from build123d import *

# Parameters (mm, degrees)
TIGE_START              = -12
ESQUISSE1_R             = 2
TIGE_DEPTH              = 12
CHANFREIN_D_ENTR_E_SIZE = 0.7
HEXAGONE_DEPTH          = 2


with BuildPart() as part:
    # Esquisse1 → Tige (new body)
    with BuildSketch(Plane(origin=(0, 0, 0), x_dir=(1, 0, 0), z_dir=(0, 1, 0)).offset(TIGE_START)):
        with Locations(Location((0, 0, 0), (0, 0, 270))):
            Circle(ESQUISSE1_R)
    extrude(amount=TIGE_DEPTH)

    # Chanfrein d'entrée
    chanfrein_d_entr_e_edges = [part.edges().sort_by_distance(p)[0] for p in [
        (0, -12, -2),
    ]]
    chamfer(chanfrein_d_entr_e_edges, length=CHANFREIN_D_ENTR_E_SIZE)

    # Esquisse2 → Tête (revolve)
    with BuildSketch(Plane.XY, mode=Mode.PRIVATE) as t_te_sk:
        with BuildLine():
            Line((1.5, 4), (1.5, 2))
            Line((1.5, 2), (0, 1.133974596))
            Line((0, 1.133974596), (0, 0))
            Line((0, 0), (3.5, 0))
            Line((3.5, 0), (3.5, 3.6))
            ThreePointArc((3.5, 3.6), (3.382842712, 3.882842712), (3.1, 4))
            Line((3.1, 4), (1.5, 4))
        make_face()
    revolve(t_te_sk.sketch.rotate(Axis((0, 4, 0), (0, -1, 0)), 180), axis=Axis((0, 4, 0), (0, -1, 0)))

    # Esquisse3 → Hexagone (cut)
    with BuildSketch(Plane(origin=(0, 4, -3), x_dir=(1, 0, 0), z_dir=(0, -1, 0))):
        Polygon((0.866025404, 4.5), (-0.866025404, 4.5), (-1.732050808, 3), (-0.866025404, 1.5), (0.866025404, 1.5), (1.732050808, 3), align=None)
    extrude(amount=HEXAGONE_DEPTH, mode=Mode.SUBTRACT)


solid = part.part
Build history of the part. All positions in model axes, mm. A direction names the side the tool comes from. Coordinates: 2 decimals unless noted, no trailing zeros. Write each loop counter-clockwise with the first axis right and the second up, starting at its lowest first coordinate (ties: lowest second). Pieces come first, ordered by that corner, then holes.
(1) 3-axis set-ups, long thin cutter, end or side, ignore diameter. For faces 5 (the flat face through (0, 3, -1.5)), 6 (the flat face through (2, 0, 2)), 7 (the flat face through (-1.3, 4, 1.3)): which of +Z, -Z, +X, -X, +Y, -Y reach the whole face in a straight line?
(2) Drill centre lines: line 1 (X direction, y = -4.75, z = -1); line 2 (Y direction, x = 2, z = 1); line 3 (Z direction, x = 0.75, y = 3.25). Where is each one in solid material? Low to high.
(3) Pin check, flat tips, straight feed: pin 1 Ø1 at (x, y) = (0, -1) entering from +Z; pin 2 Ø0.6 at (x, z) = (0.5, 1) entering from +Y; pin 3 Ø1.5 at (y, z) = (-9, 0.5) entering from +X. Stop position of each tip, or through.
(4) Cut at A-A on y = -8.5. List the corners of the cut face in (x, z).
(5) Mould opens along X. For faces 1 (the conical face through (0.19, 1.272, 0.146)), 2 (the flat face through (0, -12, 0)), 3 (the cylindrical face through (-2, -6, 0)), 4 (the flat face through (-1.293, 3.014, 0.76)) say: pulls with the +X half, pulls with the -X half, needs draft (parallel to the pull), parting line crosses it, or undercut.
Working result:
1. face 5: +Y
1. face 6: -Y
1. face 7: +Z, -Z, +X, -X, +Y
2. line 1: x = -1.73 to 1.73
2. line 2: y = 0 to 4
2. line 3: z = -3.42 to -1.5, 1.5 to 3.42
3. pin 1: stops at z = 2
3. pin 2: stops at y = 1.95
3. pin 3: stops at x = 2
4. outline: circle Ø4 at (0, 0)
5. face 1: undercut
5. face 2: needs draft
5. face 3: parting line crosses it
5. face 4: undercut
